Check sheet for the modelled part. Datum: model origin and axes. Units: mm. Give positions to 0.01 mm unless a question says otherwise; leave off trailing zeros. Order: outer loops, then holes, each group sorted by start corner. A loop starts at its lowest first (then second) coordinate and runs counter-clockwise, first axis right, second up.
Autodesk Inventor part; units mm, degrees
ref_plane "YZ Plane" through (0, 0, 0) normal (1, 0, 0) x (0, 1, 0)
ref_plane "XZ Plane" through (0, 0, 0) normal (0, 1, 0) x (-1, 0, 0)
ref_plane "XY Plane" through (0, 0, 0) normal (0, 0, 1) x (1, 0, 0)
sketch "Sketch1" plane through (0, 0, 0) normal (0, 1, 0) x (-1, 0, 0)
  line L0 (0, 0) -> (-165.1, 0)
  line L1 (-165.1, 0) -> (-165.1, -165.1)
  line L2 (-165.1, -165.1) -> (0, -165.1)
  line L3 (0, -165.1) -> (0, 0)
  circle A0 centre (-79.375, -79.375) radius 38.1
  line L4 (-25.4, -165.1) -> (-25.4, 0) construction
  line L5 (0, -25.4) -> (-165.1, -25.4) construction
  line L6 (0, 0) -> (-165.1, -165.1) construction
  circle A1 centre (-79.375, -79.375) radius 53.975 construction
  dimension "d0" = 76.2
  dimension "d3" = 25.4
  dimension "d4" = 25.4
  dimension "d5" = 107.95
  dimension "d25" = 165.1
extrude "Extrusion1" add sketch "Sketch1" along normal blind 3.175
sketch "Sketch2" plane through (0, 3.175, 0) normal (0, 1, 0) x (1, 0, 0)
  circle A0 centre (79.375, 79.375) radius 38.1 construction
  circle A1 centre (79.375, 79.375) radius 60.325 construction
  line L0 (0, 165.1) -> (0, 0) construction
  arc A2 (184.15, 82.55) -> (82.55, 184.15) centre (82.55, 82.55) ccw construction
  line L1 (36.7188, 36.7188) -> (122.0312, 36.7188) construction
  line L2 (122.0312, 36.7188) -> (122.0312, 122.0312) construction
  line L3 (122.0312, 122.0312) -> (36.7188, 122.0312) construction
  line L4 (36.7188, 122.0312) -> (36.7188, 36.7188) construction
  dimension "d9" = 120.65
hole "Hole1" at (36.7188, 3.175, -36.7188) at (122.0312, 3.175, -122.0312) at (122.0312, 3.175, -36.7188) at (36.7188, 3.175, -122.0312) direction (0, -1, 0) diameter 4.9784 end through all
sketch "Sketch3" plane through (0, 3.175, 0) normal (0, 1, 0) x (1, 0, 0)
  circle A0 centre (79.375, 79.375) radius 38.1 construction
  circle A1 centre (79.375, 79.375) radius 53.975 construction
  circle A2 centre (57.9215, 136.0171) radius 9.525
  line L0 (0, 0) -> (79.375, 79.375) construction
  circle A3 centre (136.0171, 57.9215) radius 9.525
  circle A4 centre (122.0312, 122.0312) radius 2.4892 construction
  circle A5 centre (57.9215, 136.0171) radius 22.86 construction
  line L1 (79.375, 79.375) -> (77.0039, 148.6044) construction
  circle A6 centre (77.0039, 148.6044) radius 11.1125
  circle A7 centre (148.6044, 77.0039) radius 11.1125
  circle A8 centre (57.9215, 136.0171) radius 25.4 construction
  circle A9 centre (122.0312, 122.0312) radius 4.7625 construction
  circle A10 centre (57.9215, 136.0171) radius 29.9974 construction
  circle A11 centre (36.7188, 122.0312) radius 2.4892
  circle A12 centre (43.9356, 157.2198) radius 2.4892
  circle A13 centre (122.0312, 36.7188) radius 2.4892
  circle A14 centre (157.2198, 43.9356) radius 2.4892
  circle A15 centre (71.9074, 114.8144) radius 2.4892
  circle A16 centre (114.8144, 71.9074) radius 2.4892
  circle A17 centre (79.375, 79.375) radius 38.1
  arc A18 (52.6128, 106.4932) -> (81.457, 117.4181) centre (57.9215, 136.0171) ccw
  arc A19 (117.4181, 81.457) -> (106.4932, 52.6128) centre (136.0171, 57.9215) ccw
  circle A20 centre (36.7188, 122.0312) radius 2.4892
  line L2 (36.7188, 122.0312) -> (77.0039, 148.6044) construction
  point P0 (117.4181, 81.457)
  point P1 (106.4932, 52.6128)
  dimension "d33" = 45.72
  dimension "d17" = 107.95
  dimension "d19" = 19.05
  dimension "d34" = 69.27
  dimension "d35" = 22.225
  dimension "d37" = 50.8
  dimension "d38" = 59.9948
  dimension "d39" = 9.525
  dimension "d52" = 4.9784
  dimension "d53" = 90
  dimension "d56" = 90
extrude "Extrusion5" cut sketch "Sketch3" against normal through all contours A2 | A3 | A6 | A7 | A12 | A14 | A15 A17 | A17 A15 | A17 A16 | A16 A17
extrude "Extrusion6" add sketch "Sketch3" against normal up to surface (3.175 mm away) contours A15 A17 A18 | A17 A16 A19
sketch "Sketch5" plane through (0, 3.175, 0) normal (0, 1, 0) x (1, 0, 0)
  line L0 (0, 165.1) -> (0, 0)
  line L1 (0, 0) -> (25.4, 0)
  line L2 (25.4, 0) -> (25.4, 69.85)
  line L3 (25.4, 69.85) -> (0, 69.85)
  line L4 (0, 69.85) -> (0, 0)
  line L5 (25.4, 0) -> (69.85, 0)
  line L6 (69.85, 0) -> (69.85, 25.4)
  line L7 (69.85, 25.4) -> (25.4, 25.4)
  line L8 (25.4, 25.4) -> (25.4, 0)
  dimension "d63" = 25.4
  dimension "d64" = 69.85
  dimension "d65" = 44.45
  dimension "d66" = 25.4
extrude "Extrusion7" cut sketch "Sketch5" against normal up to surface (3.175 mm away)
chamfer "Chamfer3" distance 76.2 angle 45 1 edges at (165.1, 1.5875, -165.1)
fillet "Fillet6" radius 6.35 7 edges at (165.1, 1.5875, 0) (165.1, 1.5875, -88.9) (88.9, 1.5875, -165.1) (0, 1.5875, -165.1) (25.4, 1.5875, -25.4) (0, 1.5875, -69.85) (69.85, 1.5875, 0)
sketch "Sketch6" plane through (0, 3.175, 0) normal (0, 1, 0) x (1, 0, 0)
  line L0 (0, 0) -> (12.7, 0) construction
  line L1 (12.7, 0) -> (12.7, 12.7) construction
  line L2 (12.7, 12.7) -> (0, 12.7) construction
  line L3 (0, 12.7) -> (0, 0) construction
  point P0 (25.4, 12.7)
  point P1 (38.1, 12.7)
  point P2 (50.8, 12.7)
  point P3 (63.5, 12.7)
  point P4 (76.2, 12.7)
  point P5 (88.9, 12.7)
  point P6 (101.6, 12.7)
  point P7 (114.3, 12.7)
  point P8 (127, 12.7)
  point P9 (139.7, 12.7)
  point P10 (152.4, 12.7)
  point P11 (12.7, 25.4)
  point P12 (12.7, 38.1)
  point P13 (12.7, 50.8)
  point P14 (12.7, 63.5)
  point P15 (12.7, 76.2)
  point P16 (12.7, 88.9)
  point P17 (12.7, 101.6)
  point P18 (12.7, 114.3)
  point P19 (12.7, 127)
  point P20 (12.7, 139.7)
  point P21 (12.7, 152.4)
  dimension "d77" = 12.7
  dimension "d78" = 12.7
  dimension "d81" = 12.7
  dimension "d88" = 12.7
hole "Hole2" at (12.7, 3.175, -12.7) at (25.4, 3.175, -12.7) at (38.1, 3.175, -12.7) at (50.8, 3.175, -12.7) at (63.5, 3.175, -12.7) at (76.2, 3.175, -12.7) at (88.9, 3.175, -12.7) at (101.6, 3.175, -12.7) at (114.3, 3.175, -12.7) at (127, 3.175, -12.7) at (139.7, 3.175, -12.7) at (152.4, 3.175, -12.7) at (12.7, 3.175, -25.4) at (12.7, 3.175, -38.1) at (12.7, 3.175, -50.8) at (12.7, 3.175, -63.5) at (12.7, 3.175, -76.2) at (12.7, 3.175, -88.9) at (12.7, 3.175, -101.6) at (12.7, 3.175, -114.3) at (12.7, 3.175, -127) at (12.7, 3.175, -139.7) at (12.7, 3.175, -152.4) direction (0, -1, 0) diameter 4.1402 end through all
sketch "Sketch7" plane through (0, 3.175, 0) normal (0, 1, 0) x (1, 0, 0)
  arc A0 (52.6128, 106.4932) -> (106.4932, 52.6128) centre (79.375, 79.375) ccw
  arc A1 (117.4181, 81.457) -> (81.457, 117.4181) centre (79.375, 79.375) ccw
  arc A2 (52.6128, 106.4932) -> (81.457, 117.4181) centre (57.9215, 136.0171) ccw
  arc A3 (117.4181, 81.457) -> (106.4932, 52.6128) centre (136.0171, 57.9215) ccw
  circle A4 centre (79.375, 79.375) radius 12.7
  line L0 (67.1077, 76.088) -> (76.088, 67.1077)
  line L1 (76.088, 67.1077) -> (57.3012, 48.3209)
  line L2 (57.3012, 48.3209) -> (48.3209, 57.3012)
  line L3 (48.3209, 57.3012) -> (67.1077, 76.088)
  circle A5 centre (36.7188, 36.7188) radius 2.4892
  line L4 (79.375, 79.375) -> (36.7188, 36.7188) construction
  line L5 (101.4488, 110.4291) -> (110.4291, 101.4488)
  line L6 (110.4291, 101.4488) -> (91.6423, 82.662)
  line L7 (91.6423, 82.662) -> (82.662, 91.6423)
  line L8 (82.662, 91.6423) -> (101.4488, 110.4291)
  circle A6 centre (79.375, 79.375) radius 5.1562
  circle A7 centre (74.1665, 74.1665) radius 0.7874
  point P0 (0, 0)
  point P1 (48.3209, 57.3012)
  point P2 (48.3209, 57.3012)
  point P3 (110.4291, 101.4488)
  dimension "d100" = 25.4
  dimension "d102" = 12.7
  dimension "d106" = 10.3124
  dimension "d107" = 1.5748
  dimension "d108" = 7.366
extrude "Extrusion8" add sketch "Sketch7" against normal up to surface (3.175 mm away) contours L2 A0 | L3 A4 L1 L2 | L0 A4 | A4 L7 L0 | A1 L5 | L5 L6 A4 L8 | A4 L7
fillet "Fillet7" radius 6.35 12 edges at (76.088, 1.5875, -67.1077) (67.1077, 1.5875, -76.088) (48.3209, 1.5875, -57.3012) (57.3012, 1.5875, -48.3209) (110.4291, 1.5875, -101.4488) (101.4488, 1.5875, -110.4291) (82.662, 1.5875, -91.6423) (91.6423, 1.5875, -82.662) (52.6128, 1.5875, -106.4932) (81.457, 1.5875, -117.4181) (106.4932, 1.5875, -52.6128) (117.4181, 1.5875, -81.457)
properties part number "TopPlate" material "Aluminum 6061"
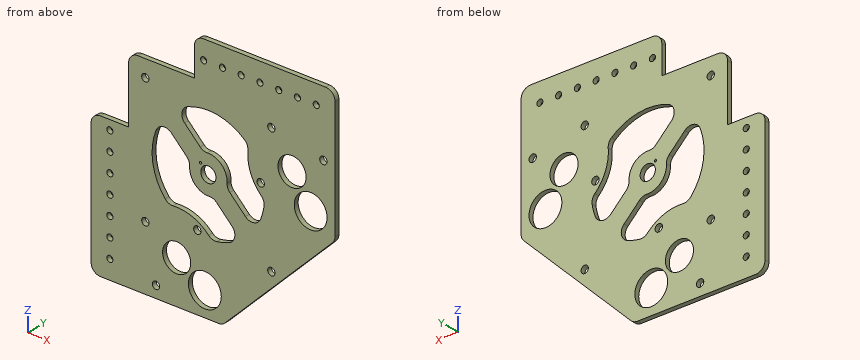
Q1. Sectioned sample at B-B, the plane z = -139.7. Record the cut outline in (x, y) (3 decimals).
Q2. Sectioned sample at C-C, the plane x = 152.4. Record the cut outline in (y, z) (3 decimals).
Q3. Sectioned sample at A-A, the plane z = -101.6. Record the cut outline in (x, y) (3 decimals).
Q4. Material ranges on line 1 (X direction, y = 0.45, z = -60.5); line 2 (X direction, y = 1.25, z = -101.5); line 3 (Z direction, x = 68.5, y = 1.15), recorded low to high.
Q5. Sectioned sample at D-D, the plane y = 1.25. Count the separate pieces of the cut face and the enclosed holes in it, plus the area to 3 significant figures.
Filled in:
1. outline: (0, 0) - (10.63, 0) - (10.63, 3.175) - (0, 3.175) - close; (14.77, 0) - (49.137, 0) - (49.137, 3.175) - (14.77, 3.175) - close; (66.706, 0) - (70.356, 0) - (70.356, 3.175) - (66.706, 3.175) - close; (83.652, 0) - (114.3, 0) - (114.3, 3.175) - (83.652, 3.175) - close
2. outline: (0, -101.6) - (3.175, -101.6) - (3.175, -87.448) - (0, -87.448) - close; (0, -66.56) - (3.175, -66.56) - (3.175, -14.77) - (0, -14.77) - close; (0, -10.63) - (3.175, -10.63) - (3.175, 0) - (0, 0) - close
3. outline: (0, 0) - (10.63, 0) - (10.63, 3.175) - (0, 3.175) - close; (14.77, 0) - (48.429, 0) - (48.429, 3.175) - (14.77, 3.175) - close; (92.62, 0) - (152.4, 0) - (152.4, 3.175) - (92.62, 3.175) - close
4. line 1: x = 25.4 to 69.48, 106.13 to 126.85, 145.19 to 165.1
4. line 2: x = 0 to 10.63, 14.77 to 48.36, 92.52 to 152.5
4. line 3: z = -165.1 to -155.76, -141.45 to -107.95, -85.93 to -59.52, -42.86 to -25.4
5. separate pieces: 1
5. enclosed holes: 30
5. area: 16,600 mm2
